For this review, use the dimensioned drawing (mm, ordinates from the lowest corner) and the shaded views. A direction names the side the tool comes from. Round coordinates to 2 decimals unless told otherwise and drop trailing zeros. Loops run counter-clockwise (first coordinate to the right, second up) from the corner with the lowest first, then second, coordinate; pieces in that order, holes last. Notation, with made-up numbers: M 78,61.25 L 103,61.25 A28 cw 103,91.25 Z; hole C -19,70.5 d7. An arc over 180 degrees is marked long. Use a Markdown table: item, result. Add a question column.
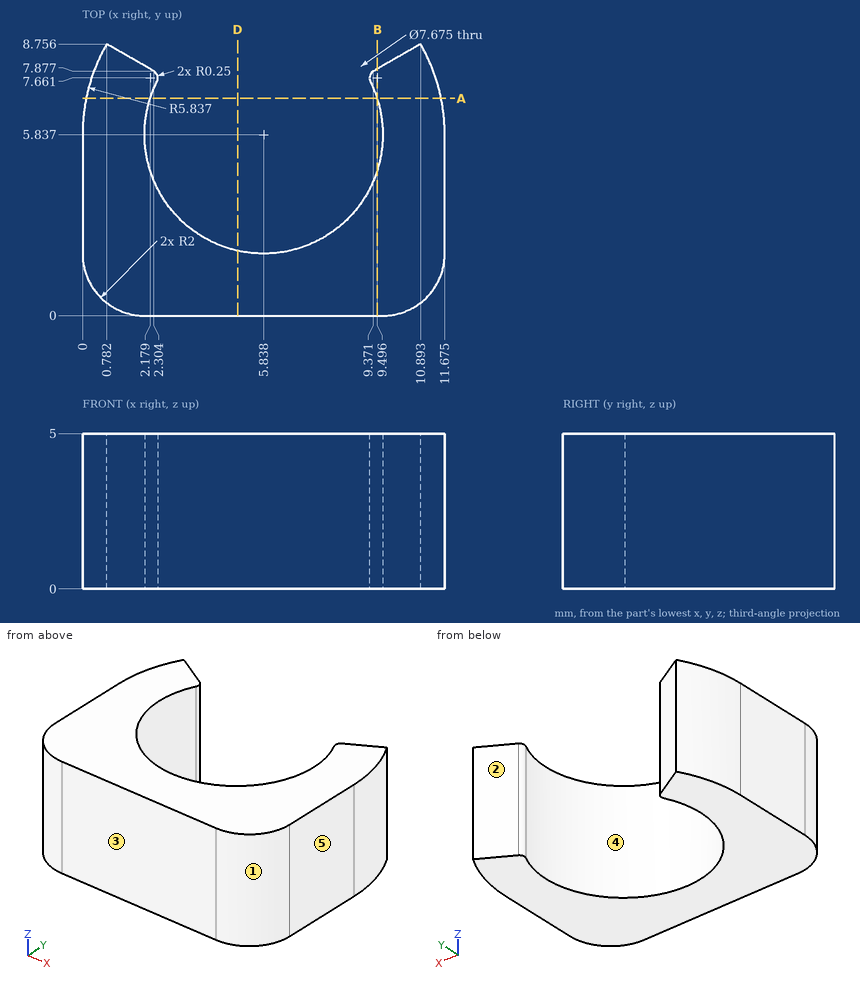
(1) Insertion check: pin 1 Ø1.5 at (y, z) = (1, 1) entering from +X; pin 2 Ø2 at (x, y) = (9, 4.5) entering from +Z. Each pin has a flat end and moves straight along its axis. Give the tip position at first contact, or say it passes through.
(2) Consider section D-D, the plane x = 5. Give the boundary of the cut face in (y, z).
(3) For the marked faces 1 and 2, list the 3-axis set-ups (+Z, -Z, +X, -X, +Y, -Y) from which the entire face can be reached by the end or side of a thin tool; tool diameter is ignored.
(4) Consider section B-B, the plane x = 9.5. Give the boundary of the cut face in (y, z).
(5) Consider section A-A, the plane y = 7. Give the boundary of the cut face in (x, z) (1 decimal).
(6) To check wall thickness, follow probe 1 along X at (y, z) = (8, 3.3) (1 decimal); probe 2 along X at (y, z) = (2.75, 1.35) (1 decimal); probe 3 along Y at (x, z) = (3.75, 3.3). State the ranges of each line that lie inside material, in increasing order.
(7) Draft analysis for pull direction X (two halves, no side actions). For the marked faces 3, 4 and 5, state which applies: released by +X, released by -X, zero draft, split by the parting line, or undercut.
Found:
| question | item | result |
|---|---|---|
| 1 | pin 1 | stops at x = 11.66 |
| 1 | pin 2 | stops at z = 5 |
| 2 | outline | M 0,0 L 2.09,0 L 2.09,5 L 0,5 Z |
| 3 | face 1 | +Z, -Z, +X, -Y |
| 3 | face 2 | +Z, -Z, +Y |
| 4 | outline | M 0,0 L 4.69,0 L 4.69,5 L 0,5 Z; M 6.98,0 L 7.95,0 L 7.95,5 L 6.98,5 Z |
| 5 | outline | M 0.1,0 L 2.2,0 L 2.2,5 L 0.1,5 Z; M 9.5,0 L 11.6,0 L 11.6,5 L 9.5,5 Z |
| 6 | probe 1 | x = 0.4 to 2.1, 9.6 to 11.3 |
| 6 | probe 2 | x = 0 to 3.6, 8.1 to 11.7 |
| 6 | probe 3 | y = 0 to 2.62 |
| 7 | face 3 | zero draft |
| 7 | face 4 | undercut |
| 7 | face 5 | released by +X |
